Source: CAD feature listing. Evaluate the final solid. Frame: model axes, mm. A direction names the side the tool comes from. Round coordinates to 2 decimals unless told otherwise and drop trailing zeros. Put each result on its own line as item: value.
```python
from build123d import *

# Parameters (mm, degrees)
CROQUIS1_W              = 7.801320344
CROQUIS1_H              = 7.801320344
CROQUIS1_R              = 2.1
SALIENTE_EXTRUIR1_DEPTH = 300
REDONDEO1_R             = 0.5


with BuildPart() as part:
    # Croquis1 → Saliente-Extruir1 (new body)
    # profile 1 of 5: a face of its own
    with BuildSketch(Plane(origin=(0, 0, 0), x_dir=(0, 0, -1), z_dir=(1, 0, 0))):
        Polygon((-6.56, 5.499339828), (-3.900660172, 2.84), (-3.900660172, 3.900660172), (-2.84, 3.900660172), (-5.499339828, 6.56), (-5.499339828, 8.2), (-3.1, 8.2), (-4.9, 10), (-10, 10), (-10, 4.9), (-8.2, 3.1), (-8.2, 5.499339828), align=None)
    # profile 2 of 5: a face of its own
    with BuildSketch(Plane(origin=(0, 0, 0), x_dir=(0, 0, -1), z_dir=(1, 0, 0))):
        Rectangle(CROQUIS1_W, CROQUIS1_H)
        Circle(CROQUIS1_R, mode=Mode.SUBTRACT)
    # profile 3 of 5: a face of its own
    with BuildSketch(Plane(origin=(0, 0, 0), x_dir=(0, 0, -1), z_dir=(1, 0, 0))):
        Polygon((5.499339828, 6.56), (2.84, 3.900660172), (3.900660172, 3.900660172), (3.900660172, 2.84), (6.56, 5.499339828), (8.2, 5.499339828), (8.2, 3.1), (10, 4.9), (10, 10), (4.9, 10), (3.1, 8.2), (5.499339828, 8.2), align=None)
    # profile 4 of 5: a face of its own
    with BuildSketch(Plane(origin=(0, 0, 0), x_dir=(0, 0, -1), z_dir=(1, 0, 0))):
        Polygon((3.900660172, -3.900660172), (2.84, -3.900660172), (5.499339828, -6.56), (5.499339828, -8.2), (3.1, -8.2), (4.9, -10), (10, -10), (10, -4.9), (8.2, -3.1), (8.2, -5.499339828), (6.56, -5.499339828), (3.900660172, -2.84), align=None)
    # profile 5 of 5: a face of its own
    with BuildSketch(Plane(origin=(0, 0, 0), x_dir=(0, 0, -1), z_dir=(1, 0, 0))):
        Polygon((-3.900660172, -3.900660172), (-3.900660172, -2.84), (-6.56, -5.499339828), (-8.2, -5.499339828), (-8.2, -3.1), (-10, -4.9), (-10, -10), (-4.9, -10), (-3.1, -8.2), (-5.499339828, -8.2), (-5.499339828, -6.56), (-2.84, -3.900660172), align=None)
    extrude(amount=SALIENTE_EXTRUIR1_DEPTH)

    # Redondeo1
    redondeo1_edges = [part.edges().sort_by_distance(p)[0] for p in [
        (150, -10, -10),
        (150, -10, 10),
        (150, 10, 10),
        (150, 10, -10),
    ]]
    fillet(redondeo1_edges, radius=REDONDEO1_R)


solid = part.part
```
Q1. Draft query along Z for faces 1 (the flat face through (148, 0, -3.901)), 2 (the flat face through (0, 2.4, 0.1)), 3 (the flat face through (148, -3.901, 0)). Return one class per face: +Z half, -Z half, draft (parallel to the pull), parting line (faces both ways), or undercut.
Ans:
face 1: -Z half
face 2: draft
face 3: undercut
Q2. Pin query (flat end, axial travel): pin 1 (8 mm diameter, centred on x = 102.5, y = 0, fed in from -Z); pin 2 (4 mm diameter, centred on x = 182.5, y = 1, fed in from +Z); pin 3 (2 mm diameter, centred on y = 5.5, z = 1, fed in from +X); pin 4 (0.7 mm diameter, centred on x = 190, z = 4, fed in from +Y). Return the tip coordinate at first contact, or that it passes through.
Ans:
pin 1: stops at z = -9.1
pin 2: stops at z = 4.06
pin 3: passes through
pin 4: stops at y = 9.45
Q3. Reachability of faces 4 (the flat face through (148, -10, -7)), 5 (the flat face through (148, 0, 3.901)), 6 (the flat face through (148, 3.901, 0)) from +Z, -Z, +X, -X, +Y, -Y: full face, straight path, thin tool, end or side. Return the list, or none.
Ans:
face 4: +Z, -Z, +X, -X, -Y
face 5: +Z, +X, -X
face 6: +X, -X, +Y
Q4. Material intervals for line 1 (Z direction, x = 196, y = -6.5); line 2 (Z direction, x = 252, y = -8), sorted ascending. Write a range as [from, to].
Ans:
line 1: z = [-10, -5.44], [5.44, 10]
line 2: z = [-10, -5.5], [5.5, 10]
